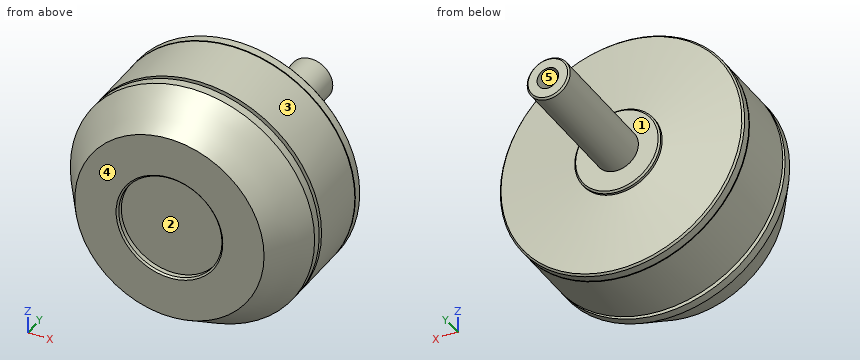
from build123d import *

# Parameters (mm, degrees)
CHAMFER_1_SIZE         = 0.2
CHAMFER_1_EDGE_2_SIZE  = 0.2
CHAMFER_1_EDGE_3_SIZE2 = 0.211806366
CHAMFER_1_EDGE_3_SIZE  = 0.2
CHAMFER_1_EDGE_4_SIZE  = 0.2
SKETCH_4_R             = 0.05


with BuildPart() as part:
    # 草图1 → 旋转1 (revolve)
    with BuildSketch(Plane.XY):
        Polygon((0, 0.750762333), (0, 19.059798334), (1.25, 19.059798334), (1.25, 31), (2.5, 31), (2.5, 16), (5, 16), (5, 15.5), (14.2, 15), (14.2, 6.5), (11, 6.5), (11, 6), (14.2, 6), (14.2, 5), (11, 0), (6, 0), (6, 0.750762333), align=None)
    revolve(axis=Axis((0, 0.750762333, 0), (0, 1, 0)))

    # 倒角1
    chamfer_1_edges = [part.edges().sort_by_distance(p)[0] for p in [
        (-2.5, 31, 0),
    ]]
    chamfer(chamfer_1_edges, length=CHAMFER_1_SIZE)

    # 倒角1 edge 2
    chamfer_1_edge_2_edges = [part.edges().sort_by_distance(p)[0] for p in [
        (-5, 16, 0),
    ]]
    chamfer(chamfer_1_edge_2_edges, length=CHAMFER_1_EDGE_2_SIZE)

    # 倒角1 edge 3
    chamfer_1_edge_3_edges = [part.edges().sort_by_distance(p)[0] for p in [
        (-14.2, 15, 0),
    ]]
    chamfer(chamfer_1_edge_3_edges, length=CHAMFER_1_EDGE_3_SIZE, length2=CHAMFER_1_EDGE_3_SIZE2)

    # 倒角1 edge 4
    chamfer_1_edge_4_edges = [part.edges().sort_by_distance(p)[0] for p in [
        (-6, 0, 0),
    ]]
    chamfer(chamfer_1_edge_4_edges, length=CHAMFER_1_EDGE_4_SIZE)

    # 草图4 → 切除-旋转4 (revolve, cut)
    with BuildSketch(Plane.XY):
        with Locations((14.193753357, 13.788193634)):
            Circle(SKETCH_4_R)
    revolve(axis=Axis((0, 32.55, 0), (0, -1, 0)), mode=Mode.SUBTRACT)


solid = part.part
For this review, take the finished solid that the model builds, in its own axes (mm). Face numbers are marked on the shaded views. A direction names the side the tool comes from. Coordinates: 2 decimals unless noted, no trailing zeros. Order: outer loops, then holes, each group sorted by start corner. A loop starts at its lowest first (then second) coordinate and runs counter-clockwise, first axis right, second up. Notation, with made-up numbers: (48.25, 67.25) - (55.25, 67.25) arc R35 cw to (55.25, 103.25) - close; hole circle Ø5 at (-17.75, 33.5). An arc over 180 degrees is marked (long way). Answer as CSV lines item,"result". Start each with the question number.
1) Draft analysis for pull direction X (two halves, no side actions). For the marked faces 1, 2 and 3, state which applies: +X half, -X half, draft (parallel to the pull), parting line (faces both ways), or undercut.
2) Add section C-C (y = 2.5). State the section outline as (x, z) points.
3) To check wall thickness, follow line 1 along Z through (x, y) = (0, 22.75); line 2 along X through (y, z) = (21.5, 1). State the ranges of each line that lie inside material, in increasing order. Write a range as [from, to].
4) Insertion check: P1, Ø6, axis at x = -2.5, z = -0.5, coming from the -Y side; P2, Ø4, axis at x = 10.5, z = 8, coming from the +Y side; P3, Ø5, axis at x = -5.5, y = 20, coming from the -Z side (3 decimals); P4, Ø2, axis at y = 19.5, z = -2.5, coming from the -X side. Each pin has a flat end and moves straight along its axis. Give the tip position at first contact, or say it passes through.
5) Add section A-A (y = 13). State the section outline as (x, z) points.
6) Add section B-B (y = 25.5). State the section outline as (x, z) points.
7) Machinability: for the marked faces 4 and 5, which of the approach directions +Z, -Z, +X, -X, +Y, -Y give a long, thin tool a straight path to every point of the face, cutting with its end or side? Answer none if there is none.
Result:
1,face 1,"draft"
1,face 2,"undercut"
1,face 3,"parting line"
2,outline,"circle Ø25.2 at (0, 0)"
3,line 1,"[-2.5, -1.25], [1.25, 2.5]"
3,line 2,"[-2.29, -0.75], [0.75, 2.29]"
4,P1,"y = 0.75"
4,P2,"y = 15.16"
4,P3,"through"
4,P4,"x = -2"
5,outline,"circle Ø28.4 at (0, 0)"
6,outline,"circle Ø5 at (0, 0); hole circle Ø2.5 at (0, 0)"
7,face 4,"+Z, -Z, +X, -X, -Y"
7,face 5,"+Y"
